Geometry check sheet. Reference: the model listing, model coordinates, mm. Give positions to 0.01 mm unless a question says otherwise; leave off trailing zeros. Loops run counter-clockwise (first coordinate to the right, second up) from the corner with the lowest first, then second, coordinate; pieces in that order, holes last. Notation, with made-up numbers: (-15.5, 42) -> (5.5, 42) arc R13 ccw to (5.5, 48) -> close; hole circle Ø7 at (-16, 10). An arc over 180 degrees is marked (long way). One line per question, with ' | ' between items.
from build123d import *

# Parameters (mm, degrees)
CYLINDER052_R          = 2
CYLINDER052_DEPTH      = 10
CYLINDER052_ROLL_ANGLE = 90
CYLINDER051_R          = 2
CYLINDER051_DEPTH      = 10
CYLINDER051_ROLL_ANGLE = 90
BOX013_W               = 16
BOX013_H               = 2
BOX013_DEPTH           = 15
CHAMFER016_SIZE        = 1


with BuildPart() as cilindro049:
    # Cylinder052 → Cylinder052 (new body)
    with BuildSketch(Plane.XY):
        Circle(CYLINDER052_R)
    extrude(amount=CYLINDER052_DEPTH)


with BuildPart() as cilindro049_1:
    # Cylinder052 roll: moved
    add(cilindro049.part.rotate(Axis((0, 0, 0), (1, 0, 0)), CYLINDER052_ROLL_ANGLE))


with BuildPart() as cilindro049_2:
    # Cylinder052 placement: moved
    add(cilindro049_1.part.moved(Location((76, -37, 30))))


with BuildPart() as fusion012:
    # Cylinder051 → Cylinder051 (new body)
    with BuildSketch(Plane.XY):
        Circle(CYLINDER051_R)
    extrude(amount=CYLINDER051_DEPTH)


with BuildPart() as fusion012_1:
    # Cylinder051 roll: moved
    add(fusion012.part.rotate(Axis((0, 0, 0), (1, 0, 0)), CYLINDER051_ROLL_ANGLE))


with BuildPart() as fusion012_2:
    # Cylinder051 placement: moved
    add(fusion012_1.part.moved(Location((67, -37, 30))))

    # Fusion012: union Cilindro049
    add(cilindro049_2.part)


with BuildPart() as obj1:
    # Box013 → Box013 (new body)
    with BuildSketch(Plane(origin=(64, -43, 23), x_dir=(1, 0, 0), z_dir=(0, 0, 1))):
        with Locations((8, 1)):
            Rectangle(BOX013_W, BOX013_H)
    extrude(amount=BOX013_DEPTH)

    # Cut040: cut Fusion012
    add(fusion012_2.part, mode=Mode.SUBTRACT)


with BuildPart() as obj1_1:
    # Cut040 placement: moved
    add(obj1.part.moved(Location((0, -7, -2))))

    # Chamfer016
    chamfer016_edges = [obj1_1.edges().sort_by_distance(p)[0] for p in [
        (72, -50, 21),
        (72, -50, 36),
    ]]
    chamfer(chamfer016_edges, length=CHAMFER016_SIZE)


solid = obj1_1.part
Item 1: Scan lines: probe 1 along X at (y, z) = (-49.55, 28); probe 2 along Z at (x, y) = (67, -48.8); probe 3 along X at (y, z) = (-48.3, 26.5). Record each from-to range of solid material in increasing order.
Result:
probe 1: 64 to 65, 69 to 74, 78 to 80 | probe 2: 21 to 26, 30 to 36 | probe 3: 64 to 65.68, 68.32 to 74.68, 77.32 to 80
Item 2: Sectioned sample at B-B (z = 28). Record the cut outline in (x, y).
Result:
outline: (64, -50) -> (65, -50) -> (65, -48) -> (64, -48) -> close; (69, -50) -> (74, -50) -> (74, -48) -> (69, -48) -> close; (78, -50) -> (80, -50) -> (80, -48) -> (78, -48) -> close
Item 3: Sectioned sample at D-D (x = 71.5). Record the cut outline in (y, z), plus the area to 3 significant figures.
Result:
outline: (-50, 22) -> (-49, 21) -> (-48, 21) -> (-48, 36) -> (-49, 36) -> (-50, 35) -> close | area: 29.0 mm2
Item 4: Depth check by flat-ended pin: pin 1 Ø3.5 at (x, z) = (76, 28) entering from +Y; pin 2 Ø6.5 at (x, z) = (67, 28) entering from -Y. Enter the tip coordinate at first touch or a pass-through.
Result:
pin 1: through | pin 2: y = -50
Item 5: Release check for a two-part mould opening along X. For faces 1 (the face through (71.9, -49.5, 35.5)), 2 (the face through (67, -49, 26)), 3 (the face through (64, -49, 28)) record: pulls with the +X half, pulls with the -X half, needs draft (parallel to the pull), parting line crosses it, or undercut.
Result:
face 1: needs draft | face 2: undercut | face 3: pulls with the -X half
Item 6: Sectioned sample at C-C (y = -49.8). Record the cut outline in (x, z), plus the area to 3 significant figures.
Result:
outline: (64, 21.8) -> (80, 21.8) -> (80, 35.2) -> (64, 35.2) -> close; hole circle Ø4 at (67, 28); hole circle Ø4 at (76, 28) | area: 189 mm2
Item 7: Sectioned sample at A-A (x = 76). Record the cut outline in (y, z), plus the area to 3 significant figures.
Result:
outline: (-50, 22) -> (-49, 21) -> (-48, 21) -> (-48, 26) -> (-50, 26) -> close; (-50, 30) -> (-48, 30) -> (-48, 36) -> (-49, 36) -> (-50, 35) -> close | area: 21.0 mm2
